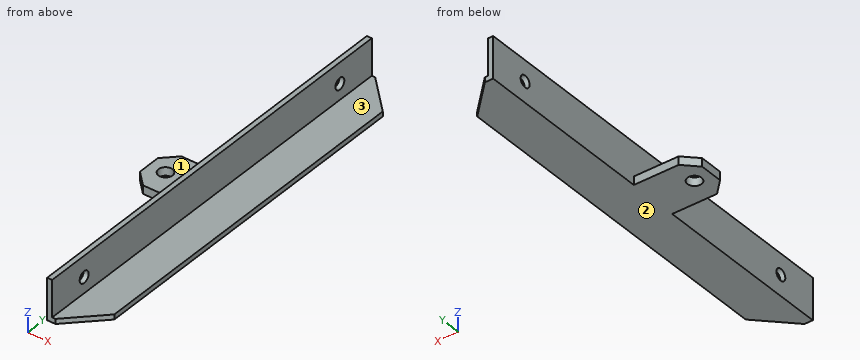
```python
from build123d import *

# Parameters (mm, degrees)
F1_DEPTH = 125
F2_SIZE  = 20
F3_W     = 35
F3_H     = 30
F3_R     = 4.25
F4_DEPTH = 5
F5_SIZE  = 8
F6_R     = 3.5
F7_DEPTH = 25


with BuildPart() as f1:
    # F0 (on Front) → F1 (new body, symmetric)
    with BuildSketch(Plane.XZ):
        Polygon((0, 25), (0, 0), (25, 0), (25, 3), (3, 3), (3, 25), align=None)
    extrude(amount=F1_DEPTH, both=True)

    # F2
    f2_edges = [f1.edges().sort_by_distance(p)[0] for p in [
        (25, -125, 1.5),
        (25, 125, 1.5),
    ]]
    chamfer(f2_edges, length=F2_SIZE)

    # F3 (on Top) → F4 (join)
    with BuildSketch(Plane.XY):
        with Locations((-17.5, 0)):
            Rectangle(F3_W, F3_H)
        with Locations((-25, 0)):
            Circle(F3_R, mode=Mode.SUBTRACT)
    extrude(amount=F4_DEPTH)

    # F5
    f5_edges = [f1.edges().sort_by_distance(p)[0] for p in [
        (-35, -15, 2.5),
        (-35, 15, 2.5),
    ]]
    chamfer(f5_edges, length=F5_SIZE)

    # F6 (on Right) → F7 (cut)
    with BuildSketch(Plane.YZ):
        with Locations((100, 12.5)):
            Circle(F6_R)
        with Locations((-100, 12.5)):
            Circle(F6_R)
    extrude(amount=F7_DEPTH, mode=Mode.SUBTRACT)


solid = f1.part
```
Work out the finished part from the listing and answer in its coordinate system (mm). Face numbers are marked on the shaded views. A direction names the side the tool comes from. Coordinates: 2 decimals unless noted, no trailing zeros. Write each loop counter-clockwise with the first axis right and the second up, starting at its lowest first coordinate (ties: lowest second). Pieces come first, ordered by that corner, then holes.
Q1. Which of the six approach directions +Z, -Z, +X, -X, +Y, -Y give full straight-line access (tool end or side, diameter ignored) to the marked faces 1, 2 and 3?
Q2. A cutting plane is placed at B-B, the plane y = 0. Give the vertices of the cut face in (x, z).
Q3. Each of these flat-tipped pins is pushed along its axis until it touches: pin 1 Ø8 at (y, z) = (47, 14.5) entering from +X; pin 2 Ø6.5 at (y, z) = (-100, 12.5) entering from -X; pin 3 Ø10 at (x, y) = (-25, 0) entering from -Z; pin 4 Ø1 at (y, z) = (-37, 3) entering from -X. Where does it stop, or does it pass through?
Q4. A cutting plane is placed at D-D, the plane y = 100. Give the vertices of the cut face in (x, z).
Q5. Find the intervals of material crossed by line 1 (Y direction, x = 2.3, z = 12.5); line 2 (Y direction, x = -25, z = 1.7); line 3 (Z direction, x = 1, y = 100), in increasing order.
Q6. A cutting plane is placed at A-A, the plane z = 12.5. Give the vertices of the cut face in (x, y).
Q7. A cutting plane is placed at C-C, the plane x = -3.5. Give the vertices of the cut face in (y, z), then the cut area to 3 significant figures.
Findings below:
1. face 1: +Z, -X, +Y, -Y
1. face 2: -Z, +X, -X, +Y, -Y
1. face 3: +Z, +X, +Y, -Y
2. outline: (-35, 0) - (-29.25, 0) - (-29.25, 5) - (-35, 5) - close; (-20.75, 0) - (25, 0) - (25, 3) - (3, 3) - (3, 25) - (0, 25) - (0, 5) - (-20.75, 5) - close
3. pin 1: stops at x = 3
3. pin 2: passes through
3. pin 3: stops at z = 0
3. pin 4: stops at x = 0
4. outline: (0, 0) - (25, 0) - (25, 3) - (3, 3) - (3, 9) - (0, 9) - close; (0, 16) - (3, 16) - (3, 25) - (0, 25) - close
5. line 1: y = -125 to -103.5, -96.5 to 96.5, 103.5 to 125
5. line 2: y = -15 to -4.25, 4.25 to 15
5. line 3: z = 0 to 9, 16 to 25
6. outline: (0, -125) - (3, -125) - (3, -103.5) - (0, -103.5) - close; (0, -96.5) - (3, -96.5) - (3, 96.5) - (0, 96.5) - close; (0, 103.5) - (3, 103.5) - (3, 125) - (0, 125) - close
7. outline: (-15, 0) - (15, 0) - (15, 5) - (-15, 5) - close
7. area: 150 mm2
